from build123d import *

# Parameters (mm, degrees)
SKETCH1_W           = 50
SKETCH1_H           = 70
BOSS_EXTRUDE1_DEPTH = 50
SKETCH2_R           = 15
BOSS_EXTRUDE2_DEPTH = 10
SKETCH3_R           = 4
BOSS_EXTRUDE3_DEPTH = 5
SHELL7_START        = 2
SHELL7_OUTLINE_W    = 46
SHELL7_OUTLINE_H    = 66
SHELL7_DEPTH        = 46
SHELL7_START_2      = 48
SHELL7_2_OUTLINE_R  = 13
SHELL7_2_DEPTH      = 10
SHELL7_START_3      = 58
SHELL7_3_OUTLINE_R  = 2
SHELL7_3_DEPTH      = 5
SKETCH4_R           = 4
BOSS_EXTRUDE4_DEPTH = 5
SCALE1_SCALE        = 0.5


# Read off the part's stored shape, not the designer's step: Shell7
with BuildPart() as part:
    # Sketch1 → Boss-Extrude1 (new body)
    with BuildSketch(Plane(origin=(0, 0, 0), x_dir=(1, 0, 0), z_dir=(0, 1, 0))):
        with Locations((25, 35)):
            Rectangle(SKETCH1_W, SKETCH1_H)
    extrude(amount=BOSS_EXTRUDE1_DEPTH)

    # Sketch2 → Boss-Extrude2 (add)
    with BuildSketch(Plane(origin=(0, 50, 0), x_dir=(1, 0, 0), z_dir=(0, 1, 0))):
        with Locations(Location((20, 20, 0), (0, 0, 90))):
            Circle(SKETCH2_R)
    extrude(amount=BOSS_EXTRUDE2_DEPTH)

    # Sketch3 → Boss-Extrude3 (add)
    with BuildSketch(Plane(origin=(0, 60, 0), x_dir=(1, 0, 0), z_dir=(0, 1, 0))):
        with Locations(Location((20, 20, 0), (0, 0, 270))):
            Circle(SKETCH3_R)
    extrude(amount=BOSS_EXTRUDE3_DEPTH)

    # Shell7 outline → Shell7 (cut)
    with BuildSketch(Plane(origin=(0, 0, 0), x_dir=(1, 0, 0), z_dir=(0, 1, 0)).offset(SHELL7_START)):
        with Locations((25, 35)):
            Rectangle(SHELL7_OUTLINE_W, SHELL7_OUTLINE_H)
    extrude(amount=SHELL7_DEPTH, mode=Mode.SUBTRACT)

    # Shell7 2 outline → Shell7 2 (cut)
    with BuildSketch(Plane(origin=(0, 0, 0), x_dir=(1, 0, 0), z_dir=(0, 1, 0)).offset(SHELL7_START_2)):
        with Locations((20, 20)):
            Circle(SHELL7_2_OUTLINE_R)
    extrude(amount=SHELL7_2_DEPTH, mode=Mode.SUBTRACT)

    # Shell7 3 outline → Shell7 3 (cut)
    with BuildSketch(Plane(origin=(0, 0, 0), x_dir=(1, 0, 0), z_dir=(0, 1, 0)).offset(SHELL7_START_3)):
        with Locations((20, 20)):
            Circle(SHELL7_3_OUTLINE_R)
    extrude(amount=SHELL7_3_DEPTH, mode=Mode.SUBTRACT)

    # Sketch4 → Boss-Extrude4 (add)
    with BuildSketch(Plane(origin=(0, 50, 0), x_dir=(1, 0, 0), z_dir=(0, 1, 0))):
        with BuildLine():
            Line((17.5, 70), (32.5, 70))
            Line((32.5, 70), (32.5, 80))
            ThreePointArc((32.5, 80), (25, 87.5), (17.5, 80))
            Line((17.5, 80), (17.5, 70))
        make_face()
        with Locations(Location((25, 80, 0), (0, 0, 270))):
            Circle(SKETCH4_R, mode=Mode.SUBTRACT)
    boss_extrude4 = extrude(amount=-BOSS_EXTRUDE4_DEPTH)

    # Mirror1: Boss-Extrude4 across plane
    add(boss_extrude4.mirror(Plane(origin=(0, 0, -35), x_dir=(1, 0, 0), z_dir=(0, 0, -1))))


with BuildPart() as part_1:
    # Scale1: scaled about (24.751384616, 27.88242139, -34.254153849)
    add(part.part.scale(SCALE1_SCALE).moved(Location((12.375692308, 13.941210695, -17.127076924))))


solid = part_1.part
Input: part model. Units: mm. Frame: model coordinates. A direction names the side the tool comes from. Round coordinates to 2 decimals unless told otherwise and drop trailing zeros. Order: outer loops, then holes, each group sorted by start corner. A loop starts at its lowest first (then second) coordinate and runs counter-clockwise, first axis right, second up.
1. Cut plane A-A, the plane y = 35.5. Output: boundary loops of the cut face in (x, z), then the cut area to 3 significant figures.
The answers:
outline: (12.38, -52.13) - (37.38, -52.13) - (37.38, -17.13) - (12.38, -17.13) - close; hole (13.38, -51.13) - (36.38, -51.13) - (36.38, -18.13) - (13.38, -18.13) - close
area: 116 mm2
2. Set-up query: faces 1 (the face through (22, 42.941, -26)), 2 (the face through (28.626, 38, -15)), 3 (the face through (24.8, 36.441, -54.6)). Return all of +Z, -Z, +X, -X, +Y, -Y with unobstructed straight access to the full face (end or side cutting, diameter ignored); none if empty.
The answers:
face 1: none
face 2: +Z, +X, +Y, -Y
face 3: -Z, +X, -X, -Y
3. Cut plane D-D, the plane z = -24. Output: boundary loops of the cut face in (x, y), then the cut area to 3 significant figures.
The answers:
outline: (12.38, 13.94) - (37.38, 13.94) - (37.38, 38.94) - (29.19, 38.94) - (29.19, 43.94) - (15.56, 43.94) - (15.56, 38.94) - (12.38, 38.94) - close; hole (13.38, 14.94) - (36.38, 14.94) - (36.38, 37.94) - (28.07, 37.94) - (28.07, 42.94) - (16.68, 42.94) - (16.68, 37.94) - (13.38, 37.94) - close
area: 107 mm2
4. Mould query, pull axis Z, two halves, no side actions, for faces 4 (the face through (24.958, 37.709, -60.876)), 5 (the face through (25, 26, -18.127)), 6 (the face through (25, 38.941, -35)). Classes: released by +Z, released by -Z, zero draft, split by the parting line, or undercut.
The answers:
face 4: released by -Z
face 5: undercut
face 6: zero draft
5. Cut plane C-C, the plane z = -53.5. Output: boundary loops of the cut face in (x, y).
The answers:
outline: (21.13, 36.44) - (28.63, 36.44) - (28.63, 38.94) - (21.13, 38.94) - close
6. Pin query (flat end, axial travel): P1, Ø2, axis at y = 37.5, z = -15, coming from the +X side; P2, Ø10, axis at x = 27.5, y = 30, coming from the +Z side; P3, Ø7.5, axis at x = 22.5, z = -35, coming from the +Y side; P4, Ø12, axis at y = 42.5, z = -30.5, coming from the +X side. Return the tip coordinate at first contact, or that it passes through.
The answers:
P1: stops at x = 28.63
P2: stops at z = -17.13
P3: stops at y = 43.94
P4: stops at x = 37.38
7. Material intervals for line 1 (X direction, y = 32, z = -49); line 2 (Y direction, x = 28.75, z = -20); line 3 (Z direction, x = 24.5, y = 16), sorted ascending.
The answers:
line 1: x = 12.38 to 13.38, 36.38 to 37.38
line 2: y = 13.94 to 14.94, 37.94 to 38.94
line 3: z = -52.13 to -51.13, -18.13 to -17.13
8. Cut plane B-B, the plane z = -37.5. Output: boundary loops of the cut face in (x, y).
The answers:
outline: (12.38, 13.94) - (37.38, 13.94) - (37.38, 38.94) - (12.38, 38.94) - close; hole (13.38, 14.94) - (36.38, 14.94) - (36.38, 37.94) - (13.38, 37.94) - close
